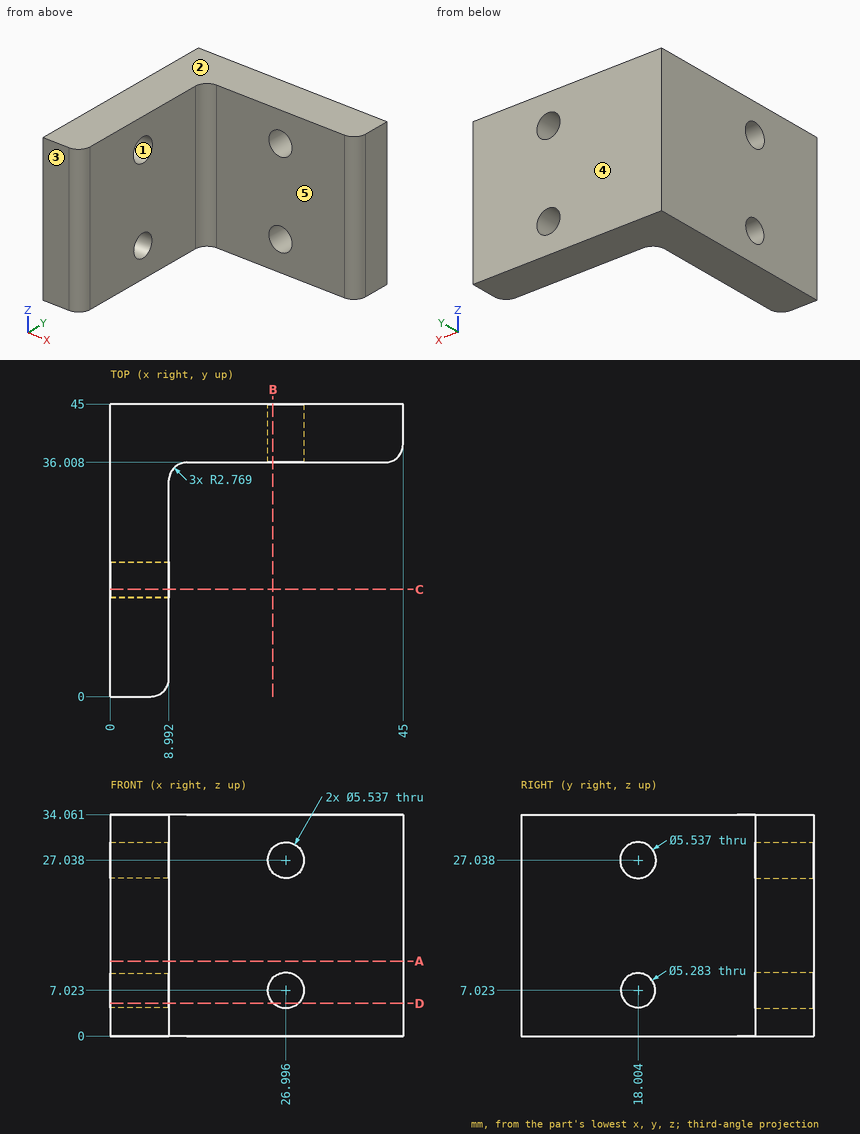
Could you check a few things on this drawing? It's one solid part, dimensions in mm from its lowest x, y, z. A direction names the side the tool comes from. Coordinates: 2 decimals unless noted, no trailing zeros. Order: outer loops, then holes, each group sorted by start corner. A loop starts at its lowest first (then second) coordinate and runs counter-clockwise, first axis right, second up. Notation, with made-up numbers: (53.25, -23) -> (76.25, -23) arc R21 cw to (76.25, -19) -> close; hole circle Ø5 at (-0.5, 72). An arc over 180 degrees is marked (long way). One line per item, written item: value. Start each with the question number.
1) Imagine slicing it at C-C on y = 16.5. List the corners of the cut face in (x, z) for me (1 decimal).
2) If I drill on L1, parallel to Z at x = 27, y = 41.5 (1 decimal); L2, parallel to Y at x = 14, z = 23; L3, parallel to X at y = 32.5, z = 12, over which ranges is the centre line in solid material (lowest first)? Write a range as [from, to].
3) Which directions (+Z, -Z, +X, -X, +Y, -Y) give clear straight access to the entire face, cutting with the end or side of a thin tool? Please do the marked faces 4 and 5.
4) I'm going to push flat-ended pins straight in: pin 1 (15 mm diameter, centred on x = 31, z = 20, fed in from -Y); pin 2 (3 mm diameter, centred on x = 8, z = 28.5, fed in from -Y); pin 3 (4 mm diameter, centred on y = 18, z = 7.02, fed in from -X); pin 4 (12 mm diameter, centred on y = 25.5, z = 17.5, fed in from +X). Where does each tip first touch, or does it pass through?
5) Imagine slicing it at D-D on z = 5. List the corners of the cut face in (x, y) for me (1 decimal).
6) We'd pull the mould along Z, two halves only. Please class the marked faces 1, 2 and 3: +Z half, -Z half, draft (parallel to the pull), parting line (faces both ways), or undercut.
7) Imagine slicing it at B-B on x = 25. List the corners of the cut face in (y, z) for me.
8) Imagine slicing it at A-A on z = 11.5. List the corners of the cut face in (x, y) for me.
Answer list:
1. outline: (0, 0) -> (9, 0) -> (9, 4.9) -> (0, 4.9) -> close; (0, 9.2) -> (9, 9.2) -> (9, 24.7) -> (0, 24.7) -> close; (0, 29.4) -> (9, 29.4) -> (9, 34.1) -> (0, 34.1) -> close
2. L1: z = [0, 4.3], [9.8, 24.3], [29.8, 34.1]
2. L2: y = [36.01, 45]
2. L3: x = [0, 8.99]
3. face 4: +Z, -Z, +X, -X, +Y
3. face 5: +Z, -Z, +X, -Y
4. pin 1: stops at y = 36.01
4. pin 2: stops at y = 0.01
4. pin 3: passes through
4. pin 4: stops at x = 8.99
5. outline: (0, 0) -> (6.2, 0) arc R2.8 ccw to (9, 2.8) -> (9, 16.3) -> (0, 16.3) -> close; (0, 19.7) -> (9, 19.7) -> (9, 33.2) arc R2.8 cw to (11.8, 36) -> (25.1, 36) -> (25.1, 45) -> (0, 45) -> close; (28.9, 36) -> (42.2, 36) arc R2.8 ccw to (45, 38.8) -> (45, 45) -> (28.9, 45) -> close
6. face 1: undercut
6. face 2: +Z half
6. face 3: draft
7. outline: (36.01, 0) -> (45, 0) -> (45, 5.1) -> (36.01, 5.1) -> close; (36.01, 8.94) -> (45, 8.94) -> (45, 25.12) -> (36.01, 25.12) -> close; (36.01, 28.96) -> (45, 28.96) -> (45, 34.06) -> (36.01, 34.06) -> close
8. outline: (0, 0) -> (6.22, 0) arc R2.77 ccw to (8.99, 2.77) -> (8.99, 33.24) arc R2.77 cw to (11.76, 36.01) -> (42.23, 36.01) arc R2.77 ccw to (45, 38.78) -> (45, 45) -> (0, 45) -> close
